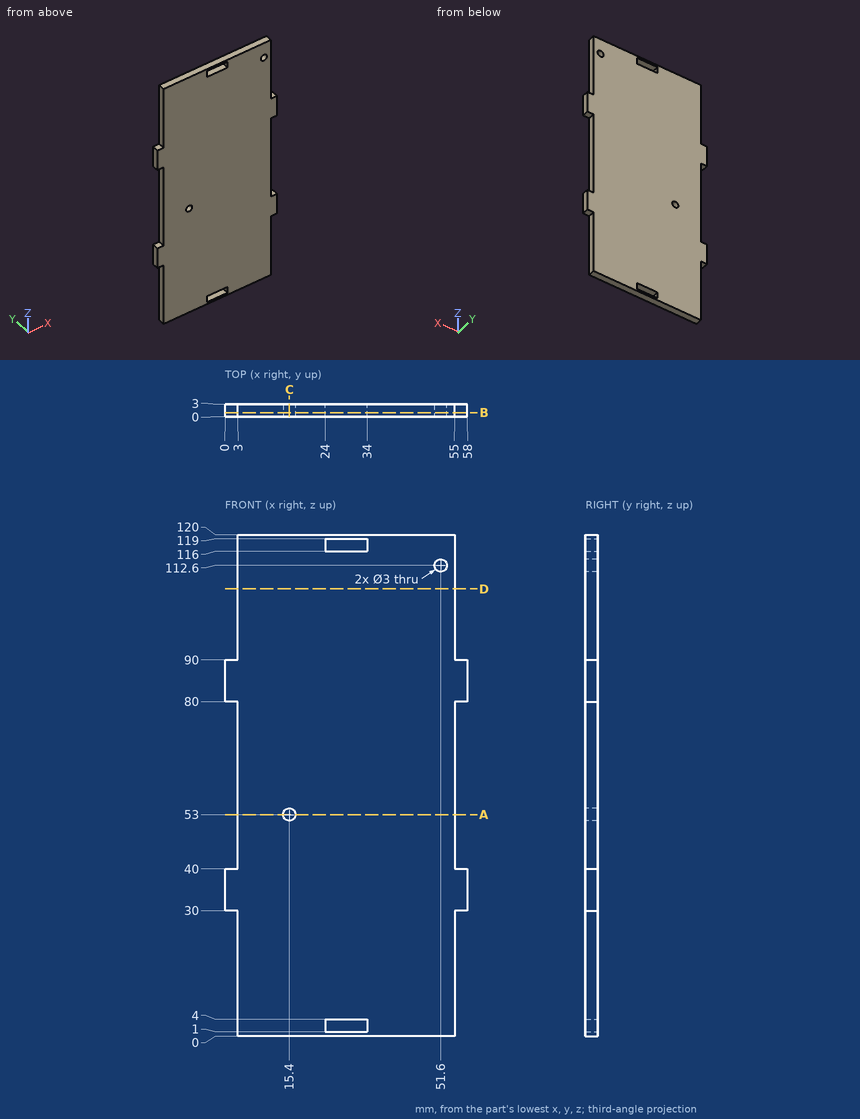
The drawing under review shows one solid part. Ordinate dimensions are in mm from its lowest x, y, z. Coordinates: 2 decimals unless noted, no trailing zeros. Order: outer loops, then holes, each group sorted by start corner. A loop starts at its lowest first (then second) coordinate and runs counter-clockwise, first axis right, second up. Notation, with made-up numbers: (46, 83.25) - (69, 83.25) arc R28 cw to (69, 122.25) - close; hole circle Ø9 at (-34.5, 76). An arc over 180 degrees is marked (long way). Put each result on its own line as item: value.
1) Take a section at D-D, the plane z = 107. Give the boundary of the cut face in (x, y), and give its area (3 significant figures).
Response values:
outline: (3, 0) - (55, 0) - (55, 3) - (3, 3) - close
area: 156 mm²
2) Wall thickness on L1, parallel to Z at x = 51.6, y = 0.85; L2, parallel to Z at x = 15.4, y = 0.6; L3, parallel to X at y = 0.8, z = 61.5: over which ranges is each line inside the solid? List them lowest first. Write a range as from..to.
Response values:
L1: z = 0..111.1, 114.1..120
L2: z = 0..51.5, 54.5..120
L3: x = 3..55
3) Insertion check: P1, Ø0.9, axis at y = 1.5, z = 118, coming from the +X side; P2, Ø1.8, axis at x = 15.4, z = 53, coming from the +Y side; P3, Ø0.9, axis at y = 2, z = 101.5, coming from the -X side; P4, Ø1.5, axis at x = 57, y = 1.5, coming from the +Z side. Each pin has a flat end and moves straight along its axis. Give the tip position at first contact, or say it passes through.
Response values:
P1: stops at x = 55
P2: passes through
P3: stops at x = 3
P4: stops at z = 90
4) Take a section at A-A, the plane z = 53. Give the boundary of the cut face in (x, y).
Response values:
outline: (3, 0) - (13.9, 0) - (13.9, 3) - (3, 3) - close; (16.9, 0) - (55, 0) - (55, 3) - (16.9, 3) - close
5) Take a section at B-B, the plane y = 0.95. Count the separate pieces of the cut face and the enclosed holes in it, and give its area (3 significant figures).
Response values:
separate pieces: 1
enclosed holes: 4
area: 6,290 mm²
6) Take a section at C-C, the plane x = 15.4. Give the boundary of the cut face in (y, z), and give its area (3 significant figures).
Response values:
outline: (0, 0) - (3, 0) - (3, 51.5) - (0, 51.5) - close; (0, 54.5) - (3, 54.5) - (3, 120) - (0, 120) - close
area: 351 mm²
